Verification items for this drawing (mm, ordinates from the low corner). Give positions to 0.01 mm unless a question says otherwise; leave off trailing zeros. Order: outer loops, then holes, each group sorted by start corner. A loop starts at its lowest first (then second) coordinate and runs counter-clockwise, first axis right, second up. Notation, with made-up numbers: M -7.75,49.25 L 7.25,49.25 A22 ccw 7.25,66.25 Z; hole C 47,37.5 d9. An arc over 180 degrees is marked long. Return JSON: item names as keys, results as strings. Group by question number.
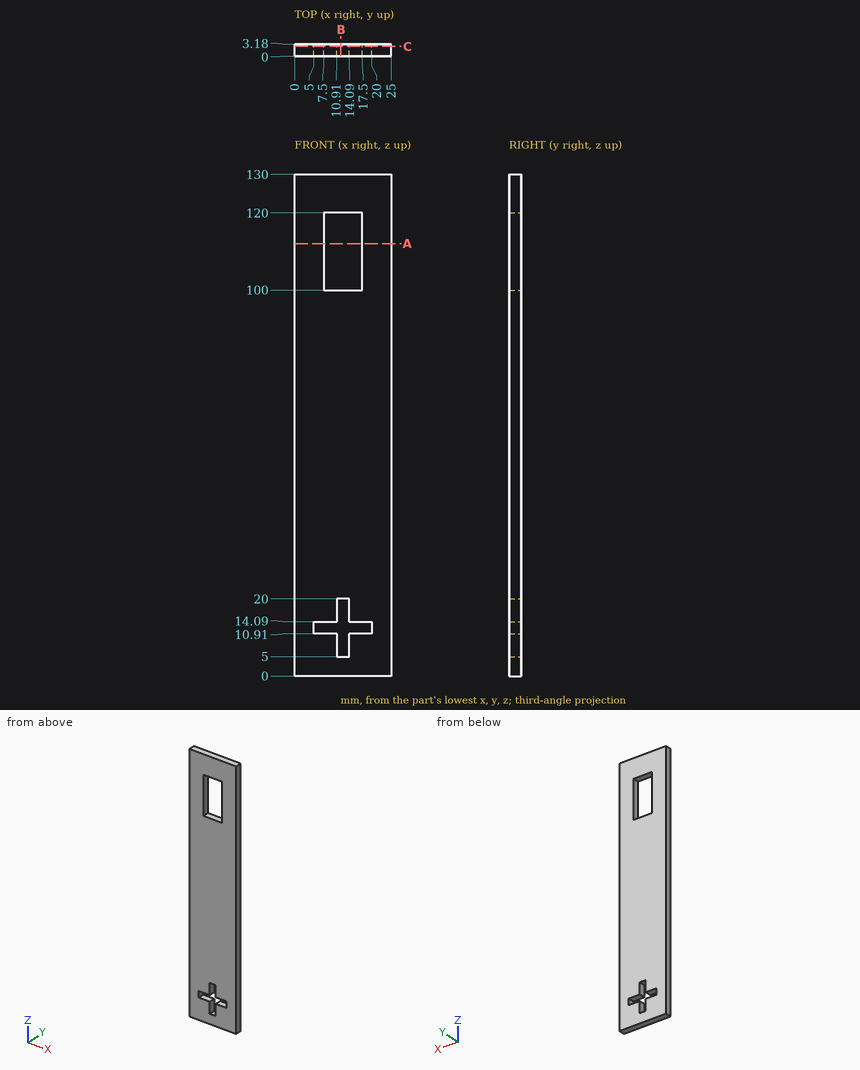
1) Sectioned sample at C-C on y = 2.55. Record the boundary of the cut face in (x, z), then the cut area to 3 significant figures.
2) Sectioned sample at B-B on x = 12. Record the boundary of the cut face in (y, z), then the cut area to 3 significant figures.
3) Sectioned sample at A-A on z = 112. Record the boundary of the cut face in (x, y), then the cut area to 3 significant figures.
4) Material ranges on line 1 along Z through (x, y) = (15, 1.85); line 2 along Z through (x, y) = (13.25, 2.55); line 3 along X through (y, z) = (0.45, 114), recorded low to high.
Reply:
{
 "1": {"outline": "M 0,0 L 25,0 L 25,130 L 0,130 Z; hole M 5,10.91 L 10.91,10.91 L 10.91,5 L 14.09,5 L 14.09,10.91 L 20,10.91 L 20,14.09 L 14.09,14.09 L 14.09,20 L 10.91,20 L 10.91,14.09 L 5,14.09 Z; hole M 7.5,100 L 17.5,100 L 17.5,120 L 7.5,120 Z", "area": "2,960 mm^2"},
 "2": {"outline": "M 0,0 L 3.18,0 L 3.18,5 L 0,5 Z; M 0,20 L 3.18,20 L 3.18,100 L 0,100 Z; M 0,120 L 3.18,120 L 3.18,130 L 0,130 Z", "area": "302 mm^2"},
 "3": {"outline": "M 0,0 L 7.5,0 L 7.5,3.18 L 0,3.18 Z; M 17.5,0 L 25,0 L 25,3.18 L 17.5,3.18 Z", "area": "47.7 mm^2"},
 "4": {"line 1": "0 to 10.91, 14.09 to 100, 120 to 130", "line 2": "0 to 5, 20 to 100, 120 to 130", "line 3": "0 to 7.5, 17.5 to 25"}
}
